Verification items for the finished model (mm, model axes). A direction names the side the tool comes from. Coordinates: 2 decimals unless noted, no trailing zeros. Write each loop counter-clockwise with the first axis right and the second up, starting at its lowest first coordinate (ties: lowest second). Pieces come first, ordered by that corner, then holes. Notation, with made-up numbers: (43, 78) -> (75, 78) arc R24 cw to (75, 99) -> close; hole circle Ø8 at (7, -35). An arc over 180 degrees is marked (long way). Write each question's results on one line, items separated by ' | '. Start each with the question number.
from build123d import *

# Parameters (mm, degrees)
BOSS_EXTRUDE1_DEPTH = 609.6
SKETCH3_R           = 4.5
CUT_EXTRUDE1_DEPTH  = 10
SKETCH6_W           = 34.925
SKETCH6_H           = 3.175
BOSS_EXTRUDE2_DEPTH = 890.4
SKETCH7_W           = 3.175
SKETCH7_H           = 38.1
BOSS_EXTRUDE3_DEPTH = 1500


with BuildPart() as part:
    # Sketch2 → Boss-Extrude1 (new body)
    with BuildSketch(Plane.XY):
        Polygon((-15.875, -15.875), (-19.05, -15.875), (-19.05, -19.05), (19.05, -19.05), (19.05, 19.05), (-19.05, 19.05), (-19.05, 15.875), (-15.875, 15.875), (15.875, 15.875), (15.875, -15.875), align=None)
    extrude(amount=BOSS_EXTRUDE1_DEPTH)

    # Sketch3 → Cut-Extrude1 (cut)
    with BuildSketch(Plane.XZ.offset(19.05)):
        with Locations(Location((0, 574.6, 0), (0, 0, 270))):
            Circle(SKETCH3_R)
        with Locations(Location((0, 539.6, 0), (0, 0, 270))):
            Circle(SKETCH3_R)
        with Locations(Location((0, 469.6, 0), (0, 0, 270))):
            Circle(SKETCH3_R)
        with Locations(Location((0, 504.6, 0), (0, 0, 270))):
            Circle(SKETCH3_R)
    extrude(amount=-CUT_EXTRUDE1_DEPTH, mode=Mode.SUBTRACT)

    # Sketch6 → Boss-Extrude2 (add)
    with BuildSketch(Plane(origin=(0, 0, 0), x_dir=(-1, 0, 0), z_dir=(0, 0, -1))):
        Polygon((19.05, -15.875), (-15.875, -15.875), (-19.05, -15.875), (-19.05, -19.05), (19.05, -19.05), align=None)
        Polygon((-15.875, 15.875), (-15.875, 19.05), (-19.05, 19.05), (-19.05, -15.875), (-15.875, -15.875), align=None)
        with Locations((1.5875, 17.4625)):
            Rectangle(SKETCH6_W, SKETCH6_H)
    extrude(amount=BOSS_EXTRUDE2_DEPTH)

    # Sketch7 → Boss-Extrude3 (add)
    with BuildSketch(Plane.XY.offset(609.6)):
        with Locations((-17.4625, 0)):
            Rectangle(SKETCH7_W, SKETCH7_H)
    extrude(amount=-BOSS_EXTRUDE3_DEPTH)


solid = part.part
1. Depth check by flat-ended pin: pin 1 Ø5.5 at (x, z) = (0, 504.6) entering from -Y (3 decimals). Enter the tip coordinate at first touch or a pass-through.
2. Sectioned sample at A-A on y = -6. Record the cut outline in (x, z) (3 decimals), plus the area to 4 significant figures.
3. Mould release check, pull along Y, two halves, no side actions. Record for faces 1 (the flat face through (-15.875, 0, -130)), 2 (the flat face through (0, -19.05, -130)), 3 (the flat face through (-17, 0, -890.4)): +Y half, -Y half, draft (parallel to the pull), parting line (faces both ways), or undercut.
4. Sectioned sample at B-B on z = 180. Record the cut outline in (x, y) (3 decimals), plus the area to 3 significant figures.
5. Material ranges on probe 1 along X at (y, z) = (-17, 469); probe 2 along Y at (x, z) = (0.5, -497.5) (3 decimals), recorded low to high. Write a range as from..to.
6. Tool access check on faces 4 (the flat face through (0, 15.875, -130)), 5 (the flat face through (-19.05, 0, -130)). Record the directions out of +Z, -Z, +X, -X, +Y, -Y that give a thin tool (end or side, any length) a straight path to the whole face; none if there is none.
Computed values:
1) pin 1: stops at y = 15.875
2) outline: (-19.05, -890.4) -> (-15.875, -890.4) -> (-15.875, 609.6) -> (-19.05, 609.6) -> close; (15.875, -890.4) -> (19.05, -890.4) -> (19.05, 609.6) -> (15.875, 609.6) -> close | area: 9,525 mm^2
3) face 1: undercut | face 2: -Y half | face 3: draft
4) outline: (-19.05, -19.05) -> (19.05, -19.05) -> (19.05, 19.05) -> (-19.05, 19.05) -> close; hole (-15.875, -15.875) -> (15.875, -15.875) -> (15.875, 15.875) -> (-15.875, 15.875) -> close | area: 444 mm^2
5) probe 1: x = -19.05..-4.46, 4.46..19.05 | probe 2: y = -19.05..-15.875, 15.875..19.05
6) face 4: +Z, -Z | face 5: +Z, -Z, -X, +Y, -Y
